```python
from build123d import *

# Parameters (mm, degrees)
F0_W     = 36
F0_H     = 20
F0_R     = 2.35
F0_R_2   = 6.2
F1_DEPTH = 3
F0_R_3   = 4.2
F2_DEPTH = 12
F3_R     = 4


with BuildPart() as f1:
    # F0 (on Top) → F1 (new body)
    with BuildSketch(Plane.XY):
        Rectangle(F0_W, F0_H)
        with Locations((-12, 0)):
            Circle(F0_R, mode=Mode.SUBTRACT)
        Circle(F0_R_2, mode=Mode.SUBTRACT)
        with Locations((12, 0)):
            Circle(F0_R, mode=Mode.SUBTRACT)
    extrude(amount=F1_DEPTH)

    # F0 (on Top) → F2 (join)
    with BuildSketch(Plane.XY):
        Circle(F0_R_2)
        Circle(F0_R_3, mode=Mode.SUBTRACT)
    extrude(amount=F2_DEPTH)

    # F3
    f3_edges = [f1.edges().sort_by_distance(p)[0] for p in [
        (-18, 10, 1.5),
        (-18, -10, 1.5),
        (18, -10, 1.5),
        (18, 10, 1.5),
    ]]
    fillet(f3_edges, radius=F3_R)


solid = f1.part
```
Geometry check sheet. Reference: the model listing, model coordinates, mm. A direction names the side the tool comes from. Coordinates: 2 decimals unless noted, no trailing zeros. Loops run counter-clockwise (first coordinate to the right, second up) from the corner with the lowest first, then second, coordinate; pieces in that order, holes last.
Item 1: Release check for a two-part mould opening along X. For faces 3 (the face through (-16.859, 8.797, 1.521)), 4 (the face through (0, 10, 1)), 5 (the face through (4.006, 1.262, 5.916)) record: released by +X, released by -X, zero draft, split by the parting line, or undercut.
Item 2: Sectioned sample at B-B, the plane x = -12. Record the boundary of the cut face in (y, z).
Item 3: Go/stop test with flat-tipped pins: pin 1 Ø8 at (x, y) = (13, 2.5) entering from +Z; pin 2 Ø1 at (y, z) = (6, 7) entering from +X; pin 3 Ø1 at (y, z) = (7, 2.5) entering from +X; pin 4 Ø5 at (x, y) = (0, 0) entering from -Z. Record where each tip stops, or that it passes through.
Item 4: Thickness scan on line 1 (Y direction, x = 0, z = 7.25); line 2 (X direction, y = 1, z = 2.75); line 3 (Z direction, x = -15, y = 4.5). Record the ranges inside material, lowest first.
Item 5: Sectioned sample at D-D, the plane x = 0. Record the boundary of the cut face in (y, z).
Item 6: Access from +Z, -Z, +X, -X, +Y, -Y to the whole of each face (thin tool, end or side, straight path). Record for faces 1 (the face through (2.86, -5.5, 7.44)), 2 (the face through (-18, 0, 1)).
Item 7: Sectioned sample at A-A, the plane y = 0. Record the boundary of the cut face in (x, z), then the cut area to 3 significant figures.
Item 8: Sectioned sample at C-C, the plane z = 8.25. Record the boundary of the cut face in (x, y), then the cut area to 3 significant figures.
Check result:
1. face 3: released by -X
1. face 4: zero draft
1. face 5: undercut
2. outline: (-10, 0) - (-2.35, 0) - (-2.35, 3) - (-10, 3) - close; (2.35, 0) - (10, 0) - (10, 3) - (2.35, 3) - close
3. pin 1: stops at z = 3
3. pin 2: stops at x = 2.86
3. pin 3: stops at x = 17.97
3. pin 4: passes through
4. line 1: y = -6.2 to -4.2, 4.2 to 6.2
4. line 2: x = -18 to -14.13, -9.87 to -4.08, 4.08 to 9.87, 14.13 to 18
4. line 3: z = 0 to 3
5. outline: (-10, 0) - (-4.2, 0) - (-4.2, 12) - (-6.2, 12) - (-6.2, 3) - (-10, 3) - close; (4.2, 0) - (10, 0) - (10, 3) - (6.2, 3) - (6.2, 12) - (4.2, 12) - close
6. face 1: +Z
6. face 2: +Z, -Z, -X, +Y, -Y
7. outline: (-18, 0) - (-14.35, 0) - (-14.35, 3) - (-18, 3) - close; (-9.65, 0) - (-4.2, 0) - (-4.2, 12) - (-6.2, 12) - (-6.2, 3) - (-9.65, 3) - close; (4.2, 0) - (9.65, 0) - (9.65, 3) - (6.2, 3) - (6.2, 12) - (4.2, 12) - close; (14.35, 0) - (18, 0) - (18, 3) - (14.35, 3) - close
7. area: 90.6 mm2
8. outline: circle Ø12.4 at (0, 0); hole circle Ø8.4 at (0, 0)
8. area: 65.3 mm2
